Could you check a few things on this model? Use its own coordinates, in mm. Coordinates: 2 decimals unless noted, no trailing zeros. Write each loop counter-clockwise with the first axis right and the second up, starting at its lowest first coordinate (ties: lowest second). Pieces come first, ordered by that corner, then holes.
Item 1: I want a section at D-D on x = 0.5. Please give me the cut outline in (y, z), then the cut area to 3 significant figures.
Item 2: I want a section at A-A on z = 0. Please give me the cut outline in (x, y).
Item 3: If I drill on probe 1 along X at (y, z) = (2.3, 0); probe 2 along X at (y, z) = (0.3, 0.6); probe 3 along Z at (x, y) = (0, 1.6), over which ranges is the centre line in solid material (lowest first)?
Item 4: I want a section at B-B on y = 1.1. Please give me the cut outline in (x, z), then the cut area to 3 significant figures.
Item 5: I want a section at C-C on x = 9. Please give me the cut outline in (y, z), then the cut area to 3 significant figures.
Item 6: Thinking about a two-plate mould opening in Z: for faces 1 (the flat face through (4, 2, -2.75)), 2 (the cylindrical face through (7.22, 1.97, 0.44)), 3 (the flat face through (4, 4, 0)), which applies, +Z half, -Z half, draft (parallel to the pull), parting line (faces both ways), or undercut?
Item 7: For P1, Ø1, axis at y = 0.5, z = -1.5, coming from the +X side; P2, Ø1, axis at x = -0.5, z = 2, coming from the -Y side, each with a flat end and sliding along its axis, tell me the tip position at first contact or that it passes through.
Autodesk Inventor part; units mm, degrees
ref_plane "YZ Plane" through (0, 0, 0) normal (1, 0, 0) x (0, 1, 0)
ref_plane "XZ Plane" through (0, 0, 0) normal (0, 1, 0) x (-1, 0, 0)
ref_plane "XY Plane" through (0, 0, 0) normal (0, 0, 1) x (1, 0, 0)
sketch "スケッチ1" plane through (0, 0, 0) normal (0, 1, 0) x (-1, 0, 0)
  circle A0 centre (0, 0) radius 1.15
  circle A1 centre (0, 0) radius 2.75
  circle A2 centre (-8.2843, 0) radius 2.75
  circle A3 centre (-8.2843, 0) radius 1.15
  line L0 (0, -2.75) -> (-8.2843, -2.75)
  line L1 (-8.2843, -2.75) -> (-8.2843, 2.75) construction
  line L2 (-8.2843, 2.75) -> (0, 2.75)
  line L3 (0, 2.75) -> (0, -2.75) construction
  line L4 (-3.55, -2.75) -> (-4.7343, -2.75)
  line L5 (-4.7343, -2.75) -> (-4.7343, 2.75)
  line L6 (-4.7343, 2.75) -> (-3.55, 2.75)
  line L7 (-3.55, 2.75) -> (-3.55, -2.75)
  circle A4 centre (0, 0) radius 3.55 construction
  circle A5 centre (-8.2843, 0) radius 3.55 construction
  circle A6 centre (-4.1421, 10) radius 10
  line L8 (0, 0) -> (-8.2843, 0)
  line L9 (-4.1421, 10) -> (0, 0)
  line L10 (-8.2843, 0) -> (-4.1421, 10)
  point P0 (-3.55, 2.75)
  point P1 (-4.7343, -2.75)
  point P2 (-8.2843, -2.75)
  point P3 (0, 2.75)
  point P4 (-4.1421, 0)
  point P5 (-4.1421, 0)
  point P6 (-4.7343, 0)
  point P7 (-3.55, 0)
  point P8 (-4.7343, 0.0175)
  point P9 (-3.55, 0.0175)
  dimension "d1" = 5.5
  dimension "d0" = 2.3
  dimension "d7" = 7.1
  dimension "d8" = 7.1
  dimension "d9" = 20
  dimension "d10" = 45
extrude "押し出し2" add sketch "スケッチ1" along normal blind 4 contours A0 A6 A1 L8 | A0 L9 A1 A6 | L8 A1 A6 A0 | A0 A6 A1 L9 | L8 L7 A6 A1 | A1 L0 L7 L8 | L9 L2 A1 | A1 A6 L7 L2 L9 | L8 A6 L7 | L7 L0 L5 L8 | A6 A3 L8 A2 | A2 L10 A3 A6 | A6 L5 L2 L7 | L8 L5 A6 | L2 L10 A2 | A2 L8 L5 L0 | A6 A2 L10 L2 L5 | L5 L8 A2 A6 | A2 A6 A3 L10 | L8 A3 A6 A2
properties part number "chain_2"
Response values:
1. outline: (0, -2.75) - (4, -2.75) - (4, -1.04) - (0, -1.04) - close; (0, 1.04) - (4, 1.04) - (4, 2.75) - (0, 2.75) - close
1. area: 13.7 mm2
2. outline: (-2.75, 0) - (-1.15, 0) - (-1.15, 4) - (-2.75, 4) - close; (1.15, 0) - (7.13, 0) - (7.13, 4) - (1.15, 4) - close; (9.43, 0) - (11.03, 0) - (11.03, 4) - (9.43, 4) - close
3. probe 1: x = -2.75 to -1.15, 1.15 to 7.13, 9.43 to 11.03
3. probe 2: x = -2.68 to -0.98, 0.98 to 7.3, 9.27 to 10.97
3. probe 3: z = -2.75 to -1.15, 1.15 to 2.75
4. outline: (0, -2.75) - (8.28, -2.75) arc R2.75 ccw to (8.28, 2.75) - (0, 2.75) arc R2.75 ccw to start; hole circle Ø2.3 at (0, 0); hole circle Ø2.3 at (8.28, 0)
4. area: 61.0 mm2
5. outline: (0, -2.66) - (4, -2.66) - (4, -0.9) - (0, -0.9) - close; (0, 0.9) - (4, 0.9) - (4, 2.66) - (0, 2.66) - close
5. area: 14.0 mm2
6. face 1: -Z half
6. face 2: undercut
6. face 3: draft
7. P1: stops at x = 10.85
7. P2: stops at y = 0
